from build123d import *

# Parameters (mm, degrees)
F0_W     = 127
F0_H     = 5.8674
F2_R     = 26.9875
F3_DEPTH = 19.05


with BuildPart() as f1:
    # F0 (on Front) → F1 (revolve)
    with BuildSketch(Plane.XZ):
        with Locations((-63.5, 27.2288)):
            Rectangle(F0_W, F0_H)
    revolve(axis=Axis((-63.5, 0, 0), (-1, 0, 0)))

    # F2 (on face) → F3 (cut)
    with BuildSketch(Plane(origin=(-127, 0, 0), x_dir=(0, -1, 0), z_dir=(-1, 0, 0))):
        Circle(F2_R)
    extrude(amount=-F3_DEPTH, mode=Mode.SUBTRACT)

    # F4: F1 across plane


with BuildPart() as f1_1:
    add(f1.part)
    add(f1.part.mirror(Plane.YZ))


solid = f1_1.part
Could you check a few things on this model? Use its own coordinates, in mm. A direction names the side the tool comes from. Round coordinates to 2 decimals unless told otherwise and drop trailing zeros. Order: outer loops, then holes, each group sorted by start corner. A loop starts at its lowest first (then second) coordinate and runs counter-clockwise, first axis right, second up.
(1) Imagine slicing it at B-B (y = 0). Write out the boundary of the cut face in (x, z), plus the area to 3 significant figures.
Response values:
outline: (-127, -30.16) - (127, -30.16) - (127, -26.99) - (107.95, -26.99) - (107.95, -24.3) - (-107.95, -24.3) - (-107.95, -26.99) - (-127, -26.99) - close; (-127, 26.99) - (-107.95, 26.99) - (-107.95, 24.3) - (107.95, 24.3) - (107.95, 26.99) - (127, 26.99) - (127, 30.16) - (-127, 30.16) - close
area: 2,780 mm2
(2) Imagine slicing it at A-A (z = 9). Write out the boundary of the cut face in (x, y), plus the area to 3 significant figures.
Response values:
outline: (-127, -28.79) - (127, -28.79) - (127, -25.44) - (107.95, -25.44) - (107.95, -22.57) - (-107.95, -22.57) - (-107.95, -25.44) - (-127, -25.44) - close; (-127, 25.44) - (-107.95, 25.44) - (-107.95, 22.57) - (107.95, 22.57) - (107.95, 25.44) - (127, 25.44) - (127, 28.79) - (-127, 28.79) - close
area: 2,940 mm2
(3) I'm going to push flat-ended pins straight in: pin 1 (8 mm diameter, centred on x = -44, y = 5.5, fed in from -Z); pin 2 (3 mm diameter, centred on y = -8.5, z = 22, fed in from +X); pin 3 (10 mm diameter, centred on x = -12, z = 9, fed in from +Y). Where does each tip first touch, or does it pass through?
Response values:
pin 1: stops at z = -30.13
pin 2: stops at x = 107.95
pin 3: stops at y = 29.9
(4) Please list where these lines run through material, in increasing order: line 1 along Y through (x, z) = (-70, 0); line 2 along Z through (x, y) = (24, 1.5); line 3 along Y through (x, z) = (85, -20.5).
Response values:
line 1: y = -30.16 to -24.3, 24.3 to 30.16
line 2: z = -30.13 to -24.25, 24.25 to 30.13
line 3: y = -22.13 to -13.04, 13.04 to 22.13
(5) If we mould it in two halves opening along Y, with no side actions, what happens to faces 3 (the flat face through (107.95, 24.1, 4.1)), 4 (the flat face through (-127, -15.5, 22.5)), 5 (the cylindrical face through (117.61, 19.89, 18.24)), 6 (the cylindrical face through (-1.778, 1.326, -30.133))? For each: released by +Y, released by -Y, zero draft, split by the parting line, or undercut.
Response values:
face 3: undercut
face 4: zero draft
face 5: undercut
face 6: split by the parting line
(6) Imagine slicing it at C-C (x = 28.5). Write out the boundary of the cut face in (y, z) (1 decimal), plus the area to 3 significant figures.
Response values:
outline: circle Ø60.3 at (0, 0); hole circle Ø48.6 at (0, 0)
area: 1,000 mm2
(7) Which directions (+Z, -Z, +X, -X, +Y, -Y) give clear straight access to the entire face, cutting with the end or side of a thin tool? Please do faces 1 (the flat face through (127, -15.5, 22.5)), 2 (the cylindrical face through (-117.61, 19.89, 18.24)).
Response values:
face 1: +Z, -Z, +X, +Y, -Y
face 2: -X
